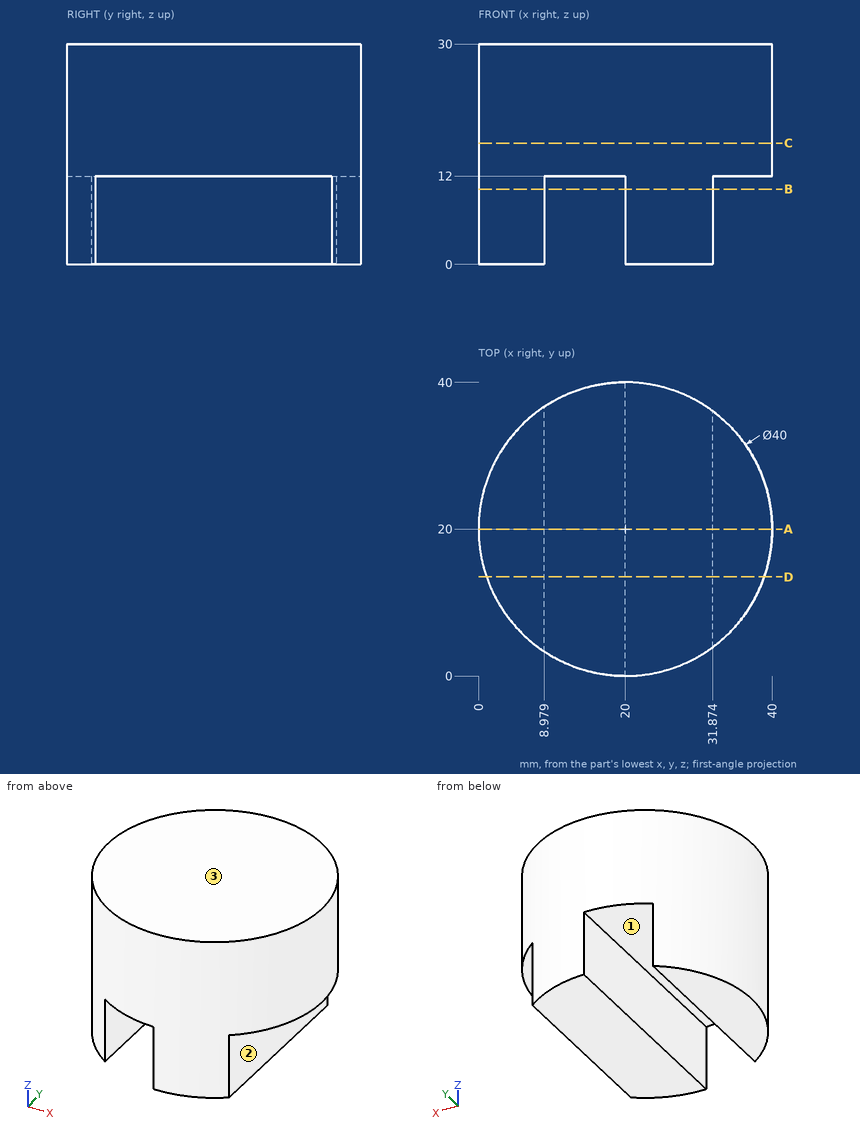
Print and shaded views of the part. All mm, measured from the part's lowest x, y and z. A direction names the side the tool comes from. Give positions to 0.01 mm unless a question says otherwise; leave off trailing zeros. Loops run counter-clockwise (first coordinate to the right, second up) from the corner with the lowest first, then second, coordinate; pieces in that order, holes last.
1) Saw through at C-C (z = 16.5). Write the cut outline in (x, y), plus the area to 3 significant figures.
2) Saw through at A-A (y = 20). Write the cut outline in (x, z).
3) Wall check: line 1 (X direction, y = 31, z = 10.5) (1 decimal); line 2 (X direction, y = 14.5, z = 7) (1 decimal); line 3 (Z direction, x = 11, y = 5). Give the ranges that are in metal, low to high.
4) Tool access for the marked faces 1, 2 and 3: list every direction of +Z, -Z, +X, -X, +Y, -Y with a clear straight run to the whole face (end or side of a thin tool).
5) Flat gauge pins, fed straight in: pin 1 Ø4 at (y, z) = (36, 16.5) entering from -X; pin 2 Ø5 at (y, z) = (17.5, 5.5) entering from -X; pin 3 Ø5 at (y, z) = (4.5, 17.5) entering from +X; pin 4 Ø13 at (y, z) = (13, 9) entering from +X. Where does each tip first touch, or does it go through?
6) Saw through at B-B (z = 10.25). Write the cut outline in (x, y), plus the area to 3 significant figures.
7) Saw through at D-D (y = 13.5). Write the cut outline in (x, z) (1 decimal), plus the area to 3 significant figures.
Answer block:
1. outline: circle Ø40 at (20, 20)
1. area: 1,260 mm2
2. outline: (0, 0) - (8.98, 0) - (8.98, 12) - (20, 12) - (20, 0) - (31.87, 0) - (31.87, 12) - (40, 12) - (40, 30) - (0, 30) - close
3. line 1: x = 3.3 to 9, 20 to 31.9
3. line 2: x = 0.8 to 9, 20 to 31.9
3. line 3: z = 12 to 30
4. face 1: -Z, +Y, -Y
4. face 2: -Z, +X, +Y, -Y
4. face 3: +Z, +X, -X, +Y, -Y
5. pin 1: stops at x = 5.72
5. pin 2: stops at x = 0
5. pin 3: stops at x = 35.2
5. pin 4: stops at x = 39.96
6. outline: (8.98, 3.31) - (8.98, 36.69) arc R20 ccw to start; (20, 0) arc R20 ccw to (31.87, 3.91) - (31.87, 36.09) arc R20 ccw to (20, 40) - close
6. area: 656 mm2
7. outline: (1.1, 0) - (9, 0) - (9, 12) - (20, 12) - (20, 0) - (31.9, 0) - (31.9, 12) - (38.9, 12) - (38.9, 30) - (1.1, 30) - close
7. area: 918 mm2
